from build123d import *

# Parameters (mm, degrees)
CUT_EXTRUDE_1_DEPTH      = 4
SKETCH_3_W               = 56
SKETCH_3_H               = 6.5
EXTRUDE_1_DEPTH          = 56
PATTERN_CIRCULAR_1_COUNT = 20


with BuildPart() as part:
    # 草图1 → 旋转2 (revolve)
    with BuildSketch(Plane.XY, mode=Mode.PRIVATE) as revolve_2_sk:
        Polygon((-56.927945362, 0), (183.072054638, 0), (183.072054638, 15), (123.072054638, 15), (123.072054638, 20), (43.072054638, 20), (43.072054638, 24), (-18.927945362, 24), (-18.927945362, 28), (-26.927945362, 28), (-26.927945362, 20), (-56.927945362, 20), align=None)
    revolve(revolve_2_sk.sketch.rotate(Axis((-87.906104207, 0, 0), (1, 0, 0)), 90), axis=Axis((-87.906104207, 0, 0), (1, 0, 0)))

    # 草图2 → 切除-拉伸1 (cut)
    with BuildSketch(Plane(origin=(0, 15, 0), x_dir=(-1, 0, 0), z_dir=(0, 1, 0))):
        with BuildLine():
            Line((-174.072054638, -4), (-132.072054638, -4))
            ThreePointArc((-132.072054638, -4), (-128.072054638, 0), (-132.072054638, 4))
            Line((-132.072054638, 4), (-174.072054638, 4))
            ThreePointArc((-174.072054638, 4), (-178.072054638, 0), (-174.072054638, -4))
        make_face()
    extrude(amount=-CUT_EXTRUDE_1_DEPTH, mode=Mode.SUBTRACT)

    # 草图3 → 旋转4 (revolve)
    with BuildSketch(Plane.XY, mode=Mode.PRIVATE) as revolve_4_sk:
        with Locations((9.072054638, 27.25)):
            Rectangle(SKETCH_3_W, SKETCH_3_H)
    revolve(revolve_4_sk.sketch.rotate(Axis((-56.927945362, 0, 0), (1, 0, 0)), 90), axis=Axis((-56.927945362, 0, 0), (1, 0, 0)))

    # 草图5 → 凸台-拉伸1 (add)
    with BuildSketch(Plane(origin=(37.072054638, 0, 0), x_dir=(0, 0, -1), z_dir=(1, 0, 0))):
        with BuildLine():
            Line((-2.63562284, 27.368933751), (2.63562284, 27.368933751))
            ThreePointArc((2.63562284, 27.368933751), (2.733180603, 31.267824503), (1.5, 34.96784237))
            Line((1.5, 34.96784237), (-1.5, 34.96784237))
            ThreePointArc((-1.5, 34.96784237), (-2.733180603, 31.267824503), (-2.63562284, 27.368933751))
        make_face()
    extrude_1 = extrude(amount=-EXTRUDE_1_DEPTH)

    # 阵列(圆周)1: 凸台-拉伸1 ×20 about axis
    pattern_circular_1_axis = Axis((0, 0, 0), (1, 0, 0))
    for i in range(1, PATTERN_CIRCULAR_1_COUNT):
        add(extrude_1.rotate(pattern_circular_1_axis, i * 360 / PATTERN_CIRCULAR_1_COUNT))


solid = part.part
Can you work these out from the model? Positions are in its coordinate system, mm. A direction names the side the tool comes from. Round coordinates to 2 decimals unless told otherwise and drop trailing zeros. Write each loop counter-clockwise with the first axis right and the second up, starting at its lowest first coordinate (ties: lowest second). Pieces come first, ordered by that corner, then holes. Notation, with made-up numbers: M 89.5,19 L 128.5,19 A11 ccw 128.5,40 Z; hole C -15,83 d2. An arc over 180 degrees is marked long. Use a Markdown table: item, result.
Item 1: If I drill on line 1 along Z through (x, y) = (19, 31); line 2 along X through (y, z) = (17, 9); line 3 along X through (y, z) = (-28.5, -5), over which ranges is the centre line in solid material (lowest first)? Write a range as [from, to].
Found:
| item | result |
|---|---|
| line 1 | z = [-12.41, -7.28], [-2.77, 2.77], [7.28, 12.41] |
| line 2 | x = [-56.93, 123.07] |
| line 3 | x = [-18.93, 37.07] |
Item 2: I want a section at A-A (x = 98.5). List the corners of the cut face in (y, z) for me, and give its area (3 significant figures).
Found:
| item | result |
|---|---|
| outline | C 0,0 d40 |
| area | 1,260 mm2 |
Item 3: Which directions (+Z, -Z, +X, -X, +Y, -Y) give clear straight access to the entire face, cutting with the end or side of a thin tool? Please do faces 5 (the face through (9.46, -32.71, 2.42)), 6 (the face through (9.46, -2.42, -32.71)), 7 (the face through (9.46, 30.43, 12.41)), 8 (the face through (9.464, 21.183, 25.037)), 9 (the face through (40.03, -7.21, 22.89)).
Found:
| item | result |
|---|---|
| face 5 | +X, -X, -Y |
| face 6 | -Z, +X, -X |
| face 7 | +X, -X |
| face 8 | +X, -X, +Y |
| face 9 | +X |
Item 4: We'd pull the mould along X, two halves only. Please class faces 1 (the face through (43.072, -20, 5)), 2 (the face through (-18.928, -26, 11)), 3 (the face through (178.07, 13.03, 0.09)), 4 (the face through (9.46, 12.41, -30.43)): released by +X, released by -X, zero draft, split by the parting line, or undercut.
Found:
| item | result |
|---|---|
| face 1 | released by +X |
| face 2 | released by -X |
| face 3 | undercut |
| face 4 | zero draft |
Item 5: For pin 1 Ø4 at (x, y) = (147, 12) entering from -Z; pin 2 Ø4 at (x, y) = (31, 13.5) entering from +Z; pin 3 Ø4 at (x, y) = (117, -15.5) entering from -Z, each with a flat end and sliding along its axis, tell me the tip position at first contact or that it passes through.
Found:
| item | result |
|---|---|
| pin 1 | stops at z = -11.18 |
| pin 2 | stops at z = 33.03 |
| pin 3 | stops at z = -14.76 |
